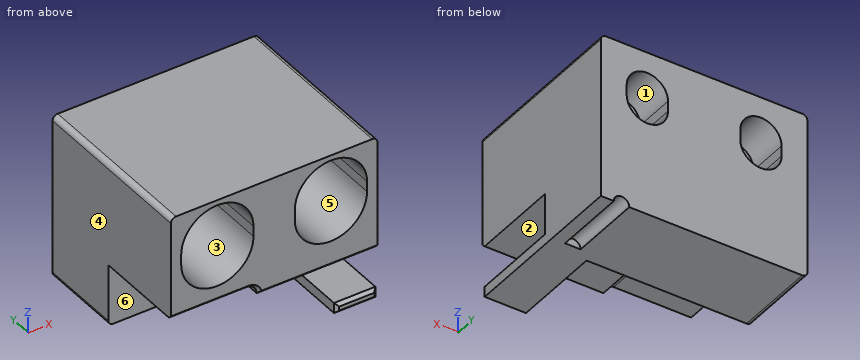
from build123d import *

# Parameters (mm, degrees)
F1_DEPTH = 17
F2_DEPTH = 8
F3_DEPTH = 17
F4_R     = 0.5
F5_DEPTH = 4
F6_SIZE  = 0.3
F7_DEPTH = 7
F8_DEPTH = 4


with BuildPart() as f1:
    # F0 (on Front) → F1 (new body)
    with BuildSketch(Plane.XZ):
        with BuildLine():
            Line((10.7877647579, 0), (10.7877647579, 11))
            Line((10.7877647579, 11), (-9.2122352421, 11))
            Line((-9.2122352421, 11), (-9.2122352421, 1.0579130137))
            ThreePointArc((-9.2122352421, 1.0579130137), (-9.2113932226, 1.0289076607), (-9.2088700001, 1))
            Line((-9.2088700001, 1), (-1.7122352421, 1))
            ThreePointArc((-1.7122352421, 1), (-1.0051284609, 0.7071067812), (-0.7122352421, 0))
            Line((-0.7122352421, 0), (0, 0))
            Line((0, 0), (10.7877647579, 0))
        make_face()
        with BuildLine():
            Line((-8.2122352421, 6), (-8.2122352421, 7))
            ThreePointArc((-8.2122352421, 7), (-4.7122352421, 10.5), (-1.2122352421, 7))
            Line((-1.2122352421, 7), (-1.2122352421, 6))
            ThreePointArc((-1.2122352421, 6), (-4.7122352421, 2.5), (-8.2122352421, 6))
        make_face(mode=Mode.SUBTRACT)
        with BuildLine():
            ThreePointArc((2.7877647579, 7), (6.2877647579, 10.5), (9.7877647579, 7))
            Line((9.7877647579, 7), (9.7877647579, 6))
            ThreePointArc((9.7877647579, 6), (6.2877647579, 2.5), (2.7877647579, 6))
            Line((2.7877647579, 6), (2.7877647579, 7))
        make_face(mode=Mode.SUBTRACT)
    extrude(amount=F1_DEPTH)

    # F0 (on Front) → F2 (join)
    with BuildSketch(Plane.XZ):
        with BuildLine():
            Line((10.7877647579, 0), (10.7877647579, 11))
            Line((10.7877647579, 11), (-9.2122352421, 11))
            Line((-9.2122352421, 11), (-9.2122352421, 1.0579130137))
            ThreePointArc((-9.2122352421, 1.0579130137), (-9.2113932226, 1.0289076607), (-9.2088700001, 1))
            Line((-9.2088700001, 1), (-1.7122352421, 1))
            ThreePointArc((-1.7122352421, 1), (-1.0051284609, 0.7071067812), (-0.7122352421, 0))
            Line((-0.7122352421, 0), (0, 0))
            Line((0, 0), (10.7877647579, 0))
        make_face()
        with BuildLine():
            Line((-8.2122352421, 6), (-8.2122352421, 7))
            ThreePointArc((-8.2122352421, 7), (-4.7122352421, 10.5), (-1.2122352421, 7))
            Line((-1.2122352421, 7), (-1.2122352421, 6))
            ThreePointArc((-1.2122352421, 6), (-4.7122352421, 2.5), (-8.2122352421, 6))
        make_face(mode=Mode.SUBTRACT)
        with BuildLine():
            ThreePointArc((2.7877647579, 7), (6.2877647579, 10.5), (9.7877647579, 7))
            Line((9.7877647579, 7), (9.7877647579, 6))
            ThreePointArc((9.7877647579, 6), (6.2877647579, 2.5), (2.7877647579, 6))
            Line((2.7877647579, 6), (2.7877647579, 7))
        make_face(mode=Mode.SUBTRACT)
        with BuildLine():
            Line((10.7877647579, -4), (10.7877647579, 0))
            Line((10.7877647579, 0), (0, 0))
            Line((0, 0), (-0.7122352421, 0))
            ThreePointArc((-0.7122352421, 0), (-1.0051284609, 0.7071067812), (-1.7122352421, 1))
            Line((-1.7122352421, 1), (-9.2088700001, 1))
            ThreePointArc((-9.2088700001, 1), (-9.2113932226, 1.0289076607), (-9.2122352421, 1.0579130137))
            Line((-9.2122352421, 1.0579130137), (-9.2122352421, -4.5))
            ThreePointArc((-9.2122352421, -4.5), (-9.0657886327, -4.8535533906), (-8.7122352421, -5))
            Line((-8.7122352421, -5), (6.7877647579, -5))
            Line((6.7877647579, -5), (6.7877647579, -4))
            Line((6.7877647579, -4), (10.7877647579, -4))
        make_face()
    extrude(amount=F2_DEPTH)

    # F0 (on Front) → F3 (join)
    with BuildSketch(Plane.XZ):
        with BuildLine():
            Line((10.7877647579, -5), (10.7877647579, -4))
            Line((10.7877647579, -4), (6.7877647579, -4))
            Line((6.7877647579, -4), (6.7877647579, -5))
            Line((6.7877647579, -5), (8.0377647579, -5))
            ThreePointArc((8.0377647579, -5), (8.7877647579, -4.25), (9.5377647579, -5))
            Line((9.5377647579, -5), (10.7877647579, -5))
        make_face()
        with BuildLine():
            Line((8.0377647579, -5), (9.5377647579, -5))
            ThreePointArc((9.5377647579, -5), (8.7877647579, -4.25), (8.0377647579, -5))
        make_face()
    extrude(amount=F3_DEPTH)

    # F4
    f4_edges = [f1.edges().sort_by_distance(p)[0] for p in [
        (-9.212235, -8.5, 11),
        (10.787765, -8.5, 11),
    ]]
    fillet(f4_edges, radius=F4_R)

    # F0 (on Front) → F5 (join)
    with BuildSketch(Plane.XZ):
        with BuildLine():
            Line((9.7877647579, 6), (9.7877647579, 7))
            ThreePointArc((9.7877647579, 7), (6.2877647579, 10.5), (2.7877647579, 7))
            Line((2.7877647579, 7), (2.7877647579, 6))
            ThreePointArc((2.7877647579, 6), (6.2877647579, 2.5), (9.7877647579, 6))
        make_face()
        with BuildLine():
            ThreePointArc((4.2877647579, 7), (6.2877647579, 9), (8.2877647579, 7))
            Line((8.2877647579, 7), (8.2877647579, 6))
            ThreePointArc((8.2877647579, 6), (6.2877647579, 4), (4.2877647579, 6))
            Line((4.2877647579, 6), (4.2877647579, 7))
        make_face(mode=Mode.SUBTRACT)
    extrude(amount=F5_DEPTH)

    # F6
    f6_edges = [f1.edges().sort_by_distance(p)[0] for p in [
        (-5.460553, -17, 1),
        (-1.005128, -17, 0.707107),
        (5.037765, -17, 0),
        (8.787765, -17, -5),
        (6.787765, -17, -4.5),
        (8.787765, -17, -4),
        (10.787765, -17, -4.5),
    ]]
    chamfer(f6_edges, length=F6_SIZE)

    # F0 (on Front) → F7 (cut)
    with BuildSketch(Plane.XZ):
        with BuildLine():
            Line((8.0377647579, -5), (9.5377647579, -5))
            ThreePointArc((9.5377647579, -5), (8.7877647579, -4.25), (8.0377647579, -5))
        make_face()
    extrude(amount=F7_DEPTH, mode=Mode.SUBTRACT)

    # F0 (on Front) → F8 (join)
    with BuildSketch(Plane.XZ):
        with BuildLine():
            ThreePointArc((-1.2122352421, 7), (-4.7122352421, 10.5), (-8.2122352421, 7))
            Line((-8.2122352421, 7), (-8.2122352421, 6))
            ThreePointArc((-8.2122352421, 6), (-4.7122352421, 2.5), (-1.2122352421, 6))
            Line((-1.2122352421, 6), (-1.2122352421, 7))
        make_face()
        with BuildLine():
            Line((-2.7122352421, 7), (-2.7122352421, 6))
            ThreePointArc((-2.7122352421, 6), (-4.7122352421, 4), (-6.7122352421, 6))
            Line((-6.7122352421, 6), (-6.7122352421, 7))
            ThreePointArc((-6.7122352421, 7), (-4.7122352421, 9), (-2.7122352421, 7))
        make_face(mode=Mode.SUBTRACT)
    extrude(amount=F8_DEPTH)


solid = f1.part
Input: part model. Units: mm. Frame: model coordinates. Face numbers are marked on the shaded views. A direction names the side the tool comes from. Round coordinates to 2 decimals unless told otherwise and drop trailing zeros. Order: outer loops, then holes, each group sorted by start corner. A loop starts at its lowest first (then second) coordinate and runs counter-clockwise, first axis right, second up. Notation, with made-up numbers: (0, 32) - (19, 32) arc R21 ccw to (19, 56) - close; hole circle Ø6 at (71, 88.5). An arc over 180 degrees is marked (long way). Answer as a JSON object with one key per item and string values. Group by question number.
(1) Cut plane B-B (y = -2.75). Return loops of the section in (x, z), then the cut area to 3 significant figures.
(2) Draft query along X for the marked faces 4, 5 and 6. Return one class per face: released by +X, released by -X, zero draft, split by the parting line, or undercut.
(3) Cut plane D-D (z = 5). Return loops of the section in (x, y), then the cut area to 3 significant figures.
(4) Cut plane A-A (y = -10.25). Return loops of the section in (x, z).
(5) Material intervals for probe 1 along X at (y, z) = (-12, 8.5); probe 2 along X at (y, z) = (-10.5, 10); probe 3 along Z at (x, y) = (9.5, -15), sorted ascending. Write a range as from..to.
(6) Pin query (flat end, axial travel): P1, Ø2, axis at x = -3.5, z = 5.5, coming from the -Y side; P2, Ø4, axis at x = 5.5, z = 9, coming from the +Y side; P3, Ø0.5, axis at y = -14, z = -4.5, coming from the -X side; P4, Ø6, axis at x = -7, y = -14.5, coming from the -Z side. Return the tip coordinate at first contact, or that it passes through.
(7) Cut plane C-C (x = 4.75). Return loops of the section in (y, z).
(8) Reachability of the marked faces 1, 2 and 3 from +Z, -Z, +X, -X, +Y, -Y: full face, straight path, thin tool, end or side. Return the list, or none.
Here are the results:
{
 "1": {"outline": "(-9.21, -4.5) arc R0.5 ccw to (-8.71, -5) - (8.04, -5) arc R0.75 cw to (9.54, -5) - (10.79, -5) - (10.79, 10.5) arc R0.5 ccw to (10.29, 11) - (-8.71, 11) arc R0.5 ccw to (-9.21, 10.5) - close; hole (-6.71, 6) arc R2 ccw to (-2.71, 6) - (-2.71, 7) arc R2 ccw to (-6.71, 7) - close; hole (4.29, 6) arc R2 ccw to (8.29, 6) - (8.29, 7) arc R2 ccw to (4.29, 7) - close", "area": "286 mm^2"},
 "2": {"face 4": "released by -X", "face 5": "undercut", "face 6": "zero draft"},
 "3": {"outline": "(-9.21, -17) - (-8.07, -17) - (-8.07, -4) - (-6.44, -4) - (-6.44, 0) - (-9.21, 0) - close; (-2.98, -4) - (-1.36, -4) - (-1.36, -17) - (2.93, -17) - (2.93, -4) - (4.56, -4) - (4.56, 0) - (-2.98, 0) - close; (8.02, -4) - (9.64, -4) - (9.64, -17) - (10.79, -17) - (10.79, 0) - (8.02, 0) - close", "area": "138 mm^2"},
 "4": {"outline": "(-9.21, 1) - (-1.71, 1) arc R1 cw to (-0.71, 0) - (10.79, 0) - (10.79, 10.5) arc R0.5 ccw to (10.29, 11) - (-8.71, 11) arc R0.5 ccw to (-9.21, 10.5) - (-9.21, 1.06) arc R0.5 ccw to start; (6.79, -5) - (10.79, -5) - (10.79, -4) - (6.79, -4) - close; hole (-8.21, 6) arc R3.5 ccw to (-1.21, 6) - (-1.21, 7) arc R3.5 ccw to (-8.21, 7) - close; hole (2.79, 6) arc R3.5 ccw to (9.79, 6) - (9.79, 7) arc R3.5 ccw to (2.79, 7) - close"},
 "5": {"probe 1": "x = -9.21..-7.87, -1.55..3.13, 9.45..10.79", "probe 2": "x = -9.21..-6.52, -2.91..4.48, 8.09..10.79", "probe 3": "z = -5..-4, 0..4.61, 8.39..11"},
 "6": {"P1": "stops at y = -4", "P2": "stops at y = 0", "P3": "stops at x = 6.79", "P4": "stops at z = 1"},
 "7": {"outline": "(-17, 0.3) - (-16.7, 0) - (-8, 0) - (-8, -5) - (0, -5) - (0, 4.72) - (-4, 4.72) - (-4, 2.86) - (-17, 2.86) - close; (-17, 10.14) - (-4, 10.14) - (-4, 8.28) - (0, 8.28) - (0, 11) - (-17, 11) - close"},
 "8": {"face 1": "+Y, -Y", "face 2": "+X, -X, -Y", "face 3": "-Y"}
}
